Geometry: final body of the model. Coordinates: model frame, mm. A direction names the side the tool comes from. Give positions to 0.01 mm unless a question says otherwise; leave off trailing zeros. Write each loop counter-clockwise with the first axis right and the second up, starting at its lowest first coordinate (ties: lowest second). Pieces come first, ordered by that corner, then holes. Notation, with made-up numbers: (6.5, 47.25) -> (27.5, 47.25) arc R21 cw to (27.5, 81.25) -> close; hole circle Ø3 at (26, 21.25). An arc over 180 degrees is marked (long way). Answer as a JSON object with one key per item and string values. Group by question number.
(1) Set-up query: faces 1 (the face through (10, -4, 5)), 2 (the face through (23, 1, 6)), 3 (the face through (0, 13, 6)), 4 (the face through (25, 5, 6)). Return all of +Z, -Z, +X, -X, +Y, -Y with unobstructed straight access to the full face (end or side cutting, diameter ignored); none if empty.
(2) Material intervals for probe 1 along X at (y, z) = (19.75, 6); probe 2 along Y at (x, z) = (3, 8.75); probe 3 along Y at (x, z) = (24, 5.5), sorted ascending.
(3) Contact query for flat-ended pins moving along their axis: pin 1 Ø5.5 at (x, z) = (-3, 7) entering from -Y; pin 2 Ø1.4 at (y, z) = (1, 9) entering from +X; pin 3 Ø3 at (y, z) = (12.5, 10) entering from -X. Output: stop coordinate, or through.
(4) Section query A-A on z = 10. Output: boundary loops of the cut face in (x, y), plus the area to 3 significant figures.
(5) Section query C-C on y = 11.75. Output: boundary loops of the cut face in (x, z).
(6) Section query B-B on x = 7.5. Output: boundary loops of the cut face in (y, z).
(7) Section query D-D on z = 6. Output: boundary loops of the cut face in (x, y).
Autodesk Inventor part; units mm, degrees
ref_plane "YZ Plane" through (0, 0, 0) normal (1, 0, 0) x (0, 1, 0)
ref_plane "XZ Plane" through (0, 0, 0) normal (0, 1, 0) x (-1, 0, 0)
ref_plane "XY Plane" through (0, 0, 0) normal (0, 0, 1) x (1, 0, 0)
sketch "Boceto1" plane through (0, 0, 0) normal (0, 0, 1) x (1, 0, 0)
  line L0 (0, 0) -> (23, 0)
  line L1 (23, 21) -> (0, 21)
  line L2 (23, 5) -> (28, 5)
  line L3 (28, 5) -> (28, 2.7)
  line L4 (28, 2.7) -> (23, 2.7)
  line L5 (0, 5) -> (-5, 5)
  line L6 (-5, 5) -> (-5, 2.7)
  line L7 (-5, 2.7) -> (0, 2.7)
  line L8 (23, 0) -> (23, 2.7)
  line L9 (23, 5) -> (23, 21)
  line L10 (0, 21) -> (0, 5)
  line L11 (0, 2.7) -> (0, 0)
  dimension "d0" = 23
  dimension "d1" = 21
  dimension "d8" = 5
  dimension "d9" = 2.3
  dimension "d10" = 5
  dimension "d11" = 2.3
extrude "Extrusión1" add sketch "Boceto1" along normal blind 12
sketch "Boceto2" plane through (0, 0, 0) normal (0, -1, 0) x (1, 0, 0)
  line L0 (0, 0) -> (0, 12)
  circle A0 centre (7.5, 6) radius 5
  dimension "d4" = 10
  dimension "d5" = 7.5
extrude "Extrusión2" add sketch "Boceto2" along normal blind 4
sketch "Boceto3" plane through (7.5, -4, 6) normal (0, -1, 0) x (1, 0, 0)
  circle A0 centre (0, 0) radius 5
  circle A1 centre (0, 0) radius 2.33
  point P0 (-7.5, -6)
  dimension "d12" = 4.66
extrude "Extrusión3" add sketch "Boceto3" along normal blind 2.7 contours A1
properties part number "Servo"
Answer list:
{
 "1": {"face 1": "-Y", "face 2": "+Z, -Z, +X, -Y", "face 3": "+Z, -Z, -X, +Y", "face 4": "+Z, -Z, +X, +Y"},
 "2": {"probe 1": "0 to 23", "probe 2": "0 to 21", "probe 3": "2.7 to 5"},
 "3": {"pin 1": "y = 2.7", "pin 2": "x = 23", "pin 3": "x = 0"},
 "4": {"outline": "(-5, 2.7) -> (0, 2.7) -> (0, 0) -> (4.5, 0) -> (4.5, -4) -> (10.5, -4) -> (10.5, 0) -> (23, 0) -> (23, 2.7) -> (28, 2.7) -> (28, 5) -> (23, 5) -> (23, 21) -> (0, 21) -> (0, 5) -> (-5, 5) -> close", "area": "530 mm2"},
 "5": {"outline": "(0, 0) -> (23, 0) -> (23, 12) -> (0, 12) -> close"},
 "6": {"outline": "(-6.7, 3.67) -> (-4, 3.67) -> (-4, 1) -> (0, 1) -> (0, 0) -> (21, 0) -> (21, 12) -> (0, 12) -> (0, 11) -> (-4, 11) -> (-4, 8.33) -> (-6.7, 8.33) -> close"},
 "7": {"outline": "(-5, 2.7) -> (0, 2.7) -> (0, 0) -> (2.5, 0) -> (2.5, -4) -> (5.17, -4) -> (5.17, -6.7) -> (9.83, -6.7) -> (9.83, -4) -> (12.5, -4) -> (12.5, 0) -> (23, 0) -> (23, 2.7) -> (28, 2.7) -> (28, 5) -> (23, 5) -> (23, 21) -> (0, 21) -> (0, 5) -> (-5, 5) -> close"}
}
